Answer from the drawing. Dimensions are ordinates in mm from the lowest x, y and z of the part. A direction names the side the tool comes from. Give positions to 0.01 mm unless a question says otherwise; leave off trailing zeros. Write each loop counter-clockwise with the first axis right and the second up, starting at its lowest first coordinate (ties: lowest second). Pieces come first, ordered by that corner, then holes.
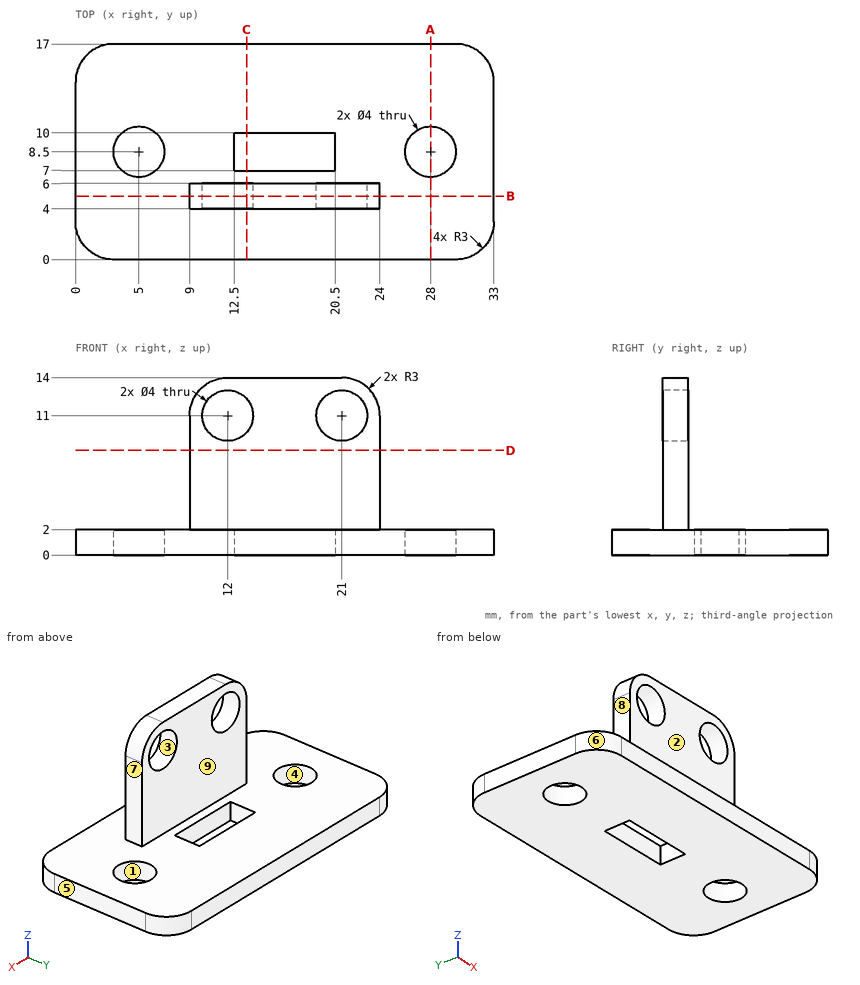
Item 1: Section B-B (y = 5) is taken. Write down the section's boundary in (x, z).
Result set:
outline: (0, 0) - (33, 0) - (33, 2) - (24, 2) - (24, 11) arc R3 ccw to (21, 14) - (12, 14) arc R3 ccw to (9, 11) - (9, 2) - (0, 2) - close; hole circle Ø4 at (12, 11); hole circle Ø4 at (21, 11)
Item 2: Determine the mould class of the marked faces 1, 2, 3 and 4 for opening direction Y: pulls with the +Y half, pulls with the -Y half, needs draft (parallel to the pull), parting line crosses it, or undercut.
Result set:
face 1: undercut
face 2: pulls with the -Y half
face 3: needs draft
face 4: undercut
Item 3: Section A-A (x = 28) is taken. Write down the section's boundary in (y, z), and give its area (3 significant figures).
Result set:
outline: (0, 0) - (6.5, 0) - (6.5, 2) - (0, 2) - close; (10.5, 0) - (17, 0) - (17, 2) - (10.5, 2) - close
area: 26.0 mm2
Item 4: Which of the six approach directions +Z, -Z, +X, -X, +Y, -Y give full straight-line access (tool end or side, diameter ignored) to the marked faces 5, 6, 7, 8 and 9?
Result set:
face 5: +Z, -Z, +X, +Y, -Y
face 6: +Z, -Z, -X, -Y
face 7: +Z, +X, +Y, -Y
face 8: +Z, -X, +Y, -Y
face 9: +Z, +X, -X, +Y
Item 5: Section D-D (z = 8.25) is taken. Write down the section's boundary in (x, y).
Result set:
outline: (9, 4) - (24, 4) - (24, 6) - (9, 6) - close
Item 6: Find the intervals of material crossed by line 1 along X through (y, z) = (5.6, 11); line 2 along Y through (x, z) = (5, 0.65); line 3 along Z through (x, y) = (11, 2), in increasing order.
Result set:
line 1: x = 9 to 10, 14 to 19, 23 to 24
line 2: y = 0 to 6.5, 10.5 to 17
line 3: z = 0 to 2
Item 7: Each of these flat-tipped pins is pushed along its axis until it touches: pin 1 Ø3.5 at (x, y) = (5, 8.5) entering from -Z (3 decimals); pin 2 Ø1.6 at (y, z) = (5.5, 8.5) entering from +X; pin 3 Ø2 at (y, z) = (4.5, 7.5) entering from -X; pin 4 Ø3.5 at (x, z) = (20, 7.5) entering from +Y. Where does it stop, or does it pass through?
Result set:
pin 1: passes through
pin 2: stops at x = 24
pin 3: stops at x = 9
pin 4: stops at y = 6
Item 8: Section C-C (x = 13.5) is taken. Write down the section's boundary in (y, z), and give its area (3 significant figures).
Result set:
outline: (0, 0) - (7, 0) - (7, 2) - (6, 2) - (6, 9.68) - (4, 9.68) - (4, 2) - (0, 2) - close; (4, 12.32) - (6, 12.32) - (6, 14) - (4, 14) - close; (10, 0) - (17, 0) - (17, 2) - (10, 2) - close
area: 46.7 mm2
